```python
from build123d import *

# Parameters (mm, degrees)
F0_R        = 3.7178453792
F1_DEPTH    = 0.889
F2_T1_DEPTH = 52.578
F3_R        = 2.54


# Not quite as in the source:
# - a fillet or chamfer that OpenCascade refuses, or shapes differently, is made with other operations: its cross-section is extruded or revolved along the edge and cut away or added


with BuildPart() as f1:
    # F0 (on Front) → F1 (new body, symmetric)
    with BuildSketch(Plane.XZ):
        with BuildLine():
            Line((19.05, -9.525), (19.05, 9.525))
            Line((19.05, 9.525), (4.9566612579, 9.525))
            ThreePointArc((4.9566612579, 9.525), (-0.016463222, 5.2090361219), (-4.9895877019, 9.525))
            Line((-4.9895877019, 9.525), (-19.05, 9.525))
            Line((-19.05, 9.525), (-19.05, -9.525))
            Line((-19.05, -9.525), (-4.9895877019, -9.525))
            ThreePointArc((-4.9895877019, -9.525), (0.067827059, -5.4479951467), (5.1252418198, -9.525))
            Line((5.1252418198, -9.525), (19.05, -9.525))
        make_face()
        Circle(F0_R, mode=Mode.SUBTRACT)
    extrude(amount=F1_DEPTH, both=True)

    # F2: fillet of radius 10.16 on 4 edges, made by hand

    # F2_s2 → F2_t1 (cut)
    with BuildSketch(Plane.XZ.offset(-26.289)):
        with BuildLine():
            ThreePointArc((-19.05, -0.635), (-16.0742048969, 6.5492048969), (-8.89, 9.525))
            Line((-8.89, 9.525), (-19.05, 9.525))
            Line((-19.05, 9.525), (-19.05, -0.635))
        make_face()
        with BuildLine():
            ThreePointArc((-8.89, -9.525), (-16.0742048969, -6.5492048969), (-19.05, 0.635))
            Line((-19.05, 0.635), (-19.05, -9.525))
            Line((-19.05, -9.525), (-8.89, -9.525))
        make_face()
        with BuildLine():
            ThreePointArc((8.89, 9.525), (16.0742048969, 6.5492048969), (19.05, -0.635))
            Line((19.05, -0.635), (19.05, 9.525))
            Line((19.05, 9.525), (8.89, 9.525))
        make_face()
        with BuildLine():
            ThreePointArc((19.05, 0.635), (16.0742048969, -6.5492048969), (8.89, -9.525))
            Line((8.89, -9.525), (19.05, -9.525))
            Line((19.05, -9.525), (19.05, 0.635))
        make_face()
    extrude(amount=F2_T1_DEPTH, mode=Mode.SUBTRACT)

    # F3
    f3_edges = [f1.edges().sort_by_distance(p)[0] for p in [
        (-4.989588, 0, 9.525),
        (5.125242, 0, -9.525),
        (-4.989588, 0, -9.525),
        (4.956661, 0, 9.525),
    ]]
    fillet(f3_edges, radius=F3_R)


solid = f1.part
```
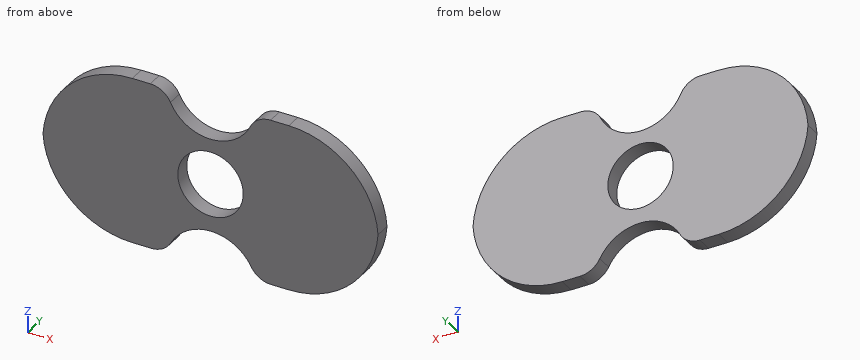
Geometry: final body of the model. Coordinates: model frame, mm. Coordinates: 2 decimals unless noted, no trailing zeros. Order: outer loops, then holes, each group sorted by start corner. A loop starts at its lowest first (then second) coordinate and runs counter-clockwise, first axis right, second up. Notation, with made-up numbers: (-14.5, 75.5) - (6.5, 75.5) arc R37 cw to (6.5, 112.5) - close; hole circle Ø6 at (46, 6.5). An arc over 180 degrees is marked (long way). Write each question's results on one line, items separated by ' | '.
(1) Section query A-A, the plane z = -7.5. Return the cut outline in (x, y), plus the area to 3 significant figures.
Values found:
outline: (-14.98, -0.89) - (-4.06, -0.89) - (-4.06, 0.89) - (-14.98, 0.89) - close; (4.19, -0.89) - (14.98, -0.89) - (14.98, 0.89) - (4.19, 0.89) - close | area: 38.6 mm²
(2) Line query: line 1 (Z direction, x = 0, y = -0.4); line 2 (X direction, y = 0.5, z = 6.5); line 3 (X direction, y = -0.6, z = -1). Output: solid intervals per line, ascending. Write a range as [from, to].
Values found:
line 1: z = [-5.45, -3.72], [3.72, 5.21] | line 2: x = [-16.12, -3.38], [3.35, 16.12] | line 3: x = [-18.92, -3.58], [3.58, 18.92]
(3) Section query B-B, the plane x = 0. Return the cut outline in (y, z).
Values found:
outline: (-0.89, -5.45) - (0.89, -5.45) - (0.89, -3.72) - (-0.89, -3.72) - close; (-0.89, 3.72) - (0.89, 3.72) - (0.89, 5.21) - (-0.89, 5.21) - close
(4) Section query C-C, the plane y = 0.6. Return the cut outline in (x, z) (3 decimals).
Values found:
outline: (-19.03, 0) arc R10.16 ccw to (-8.89, -9.525) - (-6.736, -9.525) arc R2.54 ccw to (-4.496, -8.183) arc R5.175 cw to (4.632, -8.183) arc R2.54 ccw to (6.871, -9.525) - (8.89, -9.525) arc R10.16 ccw to (19.03, 0) arc R10.16 ccw to (8.89, 9.525) - (6.814, 9.525) arc R2.54 ccw to (4.52, 8.076) arc R5.023 cw to (-4.553, 8.076) arc R2.54 ccw to (-6.847, 9.525) - (-8.89, 9.525) arc R10.16 ccw to start; hole circle Ø7.436 at (0, 0)
(5) Section query D-D, the plane x = 13. Return the cut outline in (y, z), plus the area to 3 significant figures.
Values found:
outline: (-0.89, -8.66) - (0.89, -8.66) - (0.89, 8.66) - (-0.89, 8.66) - close | area: 30.8 mm²
